```python
from build123d import *

# Parameters (mm, degrees)
SKETCH1_W               = 101.6
SKETCH1_H               = 50.8
BOSS_EXTRUDE1_DEPTH     = 304.8
CUT_EXTRUDE1_DEPTH      = 314.152231351
CUT_EXTRUDE1_DEPTH_BACK = 314.152231351
CUT_EXTRUDE2_DEPTH      = 314.152231351
CUT_EXTRUDE2_DEPTH_BACK = 314.152231351
SKETCH3_W               = 12.7
SKETCH3_H               = 304.8


with BuildPart() as part:
    # Sketch1 → Boss-Extrude1 (new body)
    with BuildSketch(Plane.XY):
        Rectangle(SKETCH1_W, SKETCH1_H)
    extrude(amount=BOSS_EXTRUDE1_DEPTH)

    # Sketch2 → Cut-Extrude1 (cut, two sides: drawn at the far end of the back side and taken through both)
    with BuildSketch(Plane(origin=(0, 25.4, 0), x_dir=(1, 0, 0), z_dir=(0, 1, 0)).offset(-CUT_EXTRUDE1_DEPTH_BACK)):
        with BuildLine():
            ThreePointArc((25.4, -298.45), (12.7, -285.75), (0, -298.45))
            ThreePointArc((0, -298.45), (0.432742006, -301.737001873), (1.701477372, -304.8))
            Line((1.701477372, -304.8), (23.698522628, -304.8))
            ThreePointArc((23.698522628, -304.8), (24.967257994, -301.737001873), (25.4, -298.45))
        make_face()
        with BuildLine():
            Line((23.698522628, -304.8), (1.701477372, -304.8))
            ThreePointArc((1.701477372, -304.8), (12.7, -311.15), (23.698522628, -304.8))
        make_face()
        with BuildLine():
            Line((25.4, -304.8), (25.4, -298.45))
            ThreePointArc((25.4, -298.45), (24.967257994, -301.737001873), (23.698522628, -304.8))
            Line((23.698522628, -304.8), (25.4, -304.8))
        make_face()
        with BuildLine():
            Line((0, -298.45), (0, -304.8))
            Line((0, -304.8), (1.701477372, -304.8))
            ThreePointArc((1.701477372, -304.8), (0.432742006, -301.737001873), (0, -298.45))
        make_face()
        Polygon((-31.75, -276.3266), (-50.8, -279.003902901), (-50.8, -304.8), (-27.748324597, -304.8), align=None)
        Polygon((-50.8, -266.17909273), (-50.8, -279.003902901), (-31.75, -276.3266), (-33.517498382, -263.750195527), align=None)
    extrude(amount=CUT_EXTRUDE1_DEPTH + CUT_EXTRUDE1_DEPTH_BACK, mode=Mode.SUBTRACT)

    # Sketch3 → Cut-Extrude2 (cut, two sides: drawn at the far end of the back side and taken through both)
    with BuildSketch(Plane(origin=(0, 25.4, 0), x_dir=(1, 0, 0), z_dir=(0, 1, 0)).offset(-CUT_EXTRUDE2_DEPTH_BACK)):
        with Locations((44.45, -152.4)):
            Rectangle(SKETCH3_W, SKETCH3_H)
    extrude(amount=CUT_EXTRUDE2_DEPTH + CUT_EXTRUDE2_DEPTH_BACK, mode=Mode.SUBTRACT)


solid = part.part
```
Read the model definition and answer for the solid it produces. Units are mm, in the model's axes. A direction names the side the tool comes from. Coordinates: 2 decimals unless noted, no trailing zeros. Loops run counter-clockwise (first coordinate to the right, second up) from the corner with the lowest first, then second, coordinate; pieces in that order, holes last.
(1) A tool of negligible diameter and unlimited length cuts with its end or side. For faces 4 (the face through (-42.038, -0.356, 264.948)), 5 (the face through (-7, 25.4, 150)), from which of +Z, -Z, +X, -X, +Y, -Y can it reach the whole face along a straight path? Write none if from no direction.
Solution:
face 4: +Z, +Y, -Y
face 5: +Z, -Z, +X, -X, +Y
(2) The part is cut by section B-B (x = 12.7). Determine the outline of the cut face in (y, z), and give its area (3 significant figures).
Solution:
outline: (-25.4, 0) - (25.4, 0) - (25.4, 285.75) - (-25.4, 285.75) - close
area: 14,500 mm2
(3) Flat-ended cylindrical pins translate along their axes: pin 1 Ø1.9 at (y, z) = (-5.5, 302) entering from -X; pin 2 Ø1.5 at (x, y) = (14.5, 18) entering from +Z. Find the tip coordinate at first contact, or state that the pin passes through.
Solution:
pin 1: stops at x = -28.28
pin 2: stops at z = 286.01
(4) The mould has two halves that part along X. Classify faces 1 (the face through (-50.8, 0, 131)), 2 (the face through (25.4, 0, 302)), 3 (the face through (32, 0, 304.8)): released by +X, released by -X, zero draft, split by the parting line, or undercut.
Solution:
face 1: released by -X
face 2: undercut
face 3: zero draft
(5) Consider line 1 along Z through (x, y) = (14, 23); line 2 along Z through (x, y) = (-43.5, -16.5). Determine where each line is inside the solid, lowest interval first.
Solution:
line 1: z = 0 to 285.82
line 2: z = 0 to 265.15
(6) The part is cut by section A-A (y = 6). Determine the outline of the cut face in (x, z), and give its area (3 significant figures).
Solution:
outline: (-50.8, 0) - (38.1, 0) - (38.1, 304.8) - (25.4, 304.8) - (25.4, 298.45) arc R12.7 cw to (0, 298.45) - (0, 304.8) - (-27.75, 304.8) - (-33.52, 263.75) - (-50.8, 266.18) - close
area: 25,900 mm2
